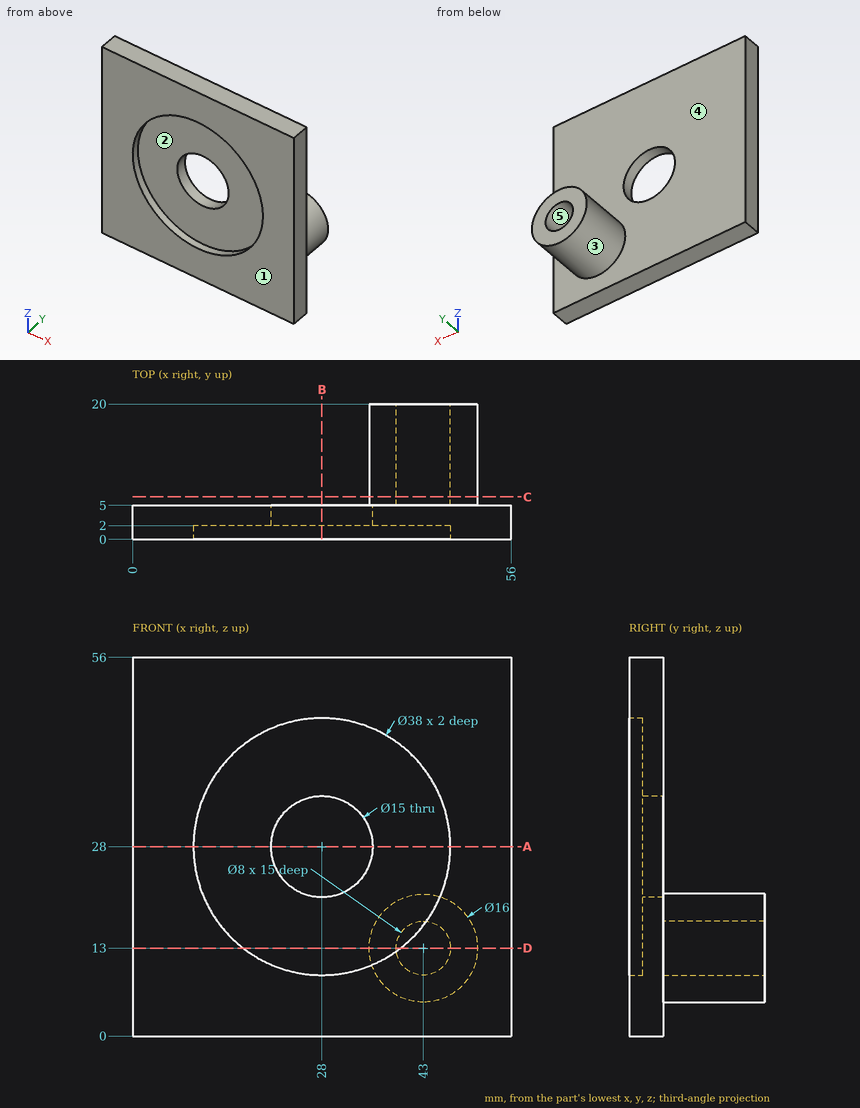
Answer from the drawing. Dimensions are ordinates in mm from the lowest x, y and z of the part. A direction names the side the tool comes from. Give positions to 0.01 mm unless a question says otherwise; leave off trailing zeros. Write each loop counter-clockwise with the first axis right and the second up, starting at its lowest first coordinate (ties: lowest second). Pieces come first, ordered by that corner, then holes. Notation, with made-up numbers: (40.25, 3) -> (46.25, 3) arc R27 ccw to (46.25, 31) -> close; hole circle Ø9 at (6, 48.25). An arc over 180 degrees is marked (long way). Use a Markdown table: item, result.
(1) Section D-D, the plane z = 13 is taken. Determine the outline of the cut face in (x, y), then the cut area to 3 significant figures.
Return value:
| item | result |
|---|---|
| outline | (0, 0) -> (16.34, 0) -> (16.34, 2) -> (39.66, 2) -> (39.66, 0) -> (56, 0) -> (56, 5) -> (51, 5) -> (51, 20) -> (47, 20) -> (47, 5) -> (39, 5) -> (39, 20) -> (35, 20) -> (35, 5) -> (0, 5) -> close |
| area | 353 mm2 |
(2) Section C-C, the plane y = 6.25 is taken. Determine the outline of the cut face in (x, z).
Return value:
| item | result |
|---|---|
| outline | circle Ø16 at (43, 13); hole circle Ø8 at (43, 13) |
(3) Determine the mould class of the marked faces 3, 4 and 5 for opening direction Z: released by +Z, released by -Z, zero draft, split by the parting line, or undercut.
Return value:
| item | result |
|---|---|
| face 3 | split by the parting line |
| face 4 | zero draft |
| face 5 | undercut |
(4) Section A-A, the plane z = 28 is taken. Determine the outline of the cut face in (x, y), then the cut area to 3 significant figures.
Return value:
| item | result |
|---|---|
| outline | (0, 0) -> (9, 0) -> (9, 2) -> (20.5, 2) -> (20.5, 5) -> (0, 5) -> close; (35.5, 2) -> (47, 2) -> (47, 0) -> (56, 0) -> (56, 5) -> (35.5, 5) -> close |
| area | 159 mm2 |
(5) For the marked faces 1 and 2, determine the directions among +Z, -Z, +X, -X, +Y, -Y from which every point of the face is accessible in a straight line to the end or side of a thin tool.
Return value:
| item | result |
|---|---|
| face 1 | +Z, -Z, +X, -X, -Y |
| face 2 | -Y |
(6) Find the intervals of material crossed by probe 1 along X at (y, z) = (8.75, 13); probe 2 along X at (y, z) = (0.6, 28); probe 3 along Y at (x, z) = (5, 18), in increasing order. Write a range as from..to.
Return value:
| item | result |
|---|---|
| probe 1 | 35..39, 47..51 |
| probe 2 | 0..9, 47..56 |
| probe 3 | 0..5 |
(7) Section B-B, the plane x = 28 is taken. Determine the outline of the cut face in (y, z).
Return value:
| item | result |
|---|---|
| outline | (0, 0) -> (5, 0) -> (5, 20.5) -> (2, 20.5) -> (2, 9) -> (0, 9) -> close; (0, 47) -> (2, 47) -> (2, 35.5) -> (5, 35.5) -> (5, 56) -> (0, 56) -> close |
(8) Flat-ended cylindrical pins translate along their axes: P1, Ø23, axis at x = 28, z = 28, coming from the -Y side; P2, Ø7, axis at x = 43, z = 13, coming from the +Y side; P3, Ø10, axis at y = 13.5, z = 25, coming from the -X side. Find the tip coordinate at first contact, or state that the pin passes through.
Return value:
| item | result |
|---|---|
| P1 | y = 2 |
| P2 | y = 5 |
| P3 | x = 39.13 |
